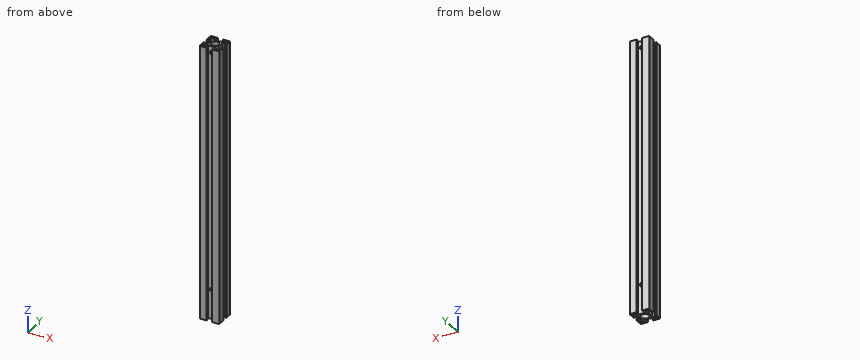
from build123d import *

# Parameters (mm, degrees)
SKETCH006_R     = 6
SKETCH006_W     = 2.75
SKETCH006_H     = 2.75
PAD_DEPTH       = 420
SKETCH_R        = 3.175
POCKET_DEPTH    = 23.250999
SKETCH007_R     = 3.175
POCKET001_DEPTH = 23.251


with BuildPart() as part:
    # Sketch006 → Pad (new body)
    with BuildSketch(Plane.XY):
        with BuildLine():
            Line((4.1, -15), (14, -15))
            ThreePointArc((14, -15), (14.707107, -14.707107), (15, -14))
            Line((15, -14), (15, -4.1))
            Line((15, -4.1), (13, -4.1))
            Line((13, -4.1), (13, -8.75))
            Line((13, -8.75), (11, -8.75))
            Line((11, -8.75), (8.249999, -6))
            Line((8.249999, -6), (8.249999, 6))
            Line((8.249999, 6), (11, 8.75))
            Line((11, 8.75), (13, 8.75))
            Line((13, 8.75), (13, 4.1))
            Line((13, 4.1), (15, 4.1))
            Line((15, 4.1), (15, 14))
            ThreePointArc((15, 14), (14.707107, 14.707107), (14.000001, 15))
            Line((14.000001, 15), (4.1, 15))
            Line((4.1, 15), (4.1, 13))
            Line((4.1, 13), (8.75, 13))
            Line((8.75, 13), (8.75, 11))
            Line((8.75, 11), (6, 8.25))
            Line((6, 8.25), (-6, 8.25))
            Line((-6, 8.25), (-8.75, 11))
            Line((-8.75, 11), (-8.75, 13))
            Line((-8.75, 13), (-4.1, 13))
            Line((-4.1, 13), (-4.1, 15))
            Line((-4.1, 15), (-14, 15))
            ThreePointArc((-14, 15), (-14.707107, 14.707107), (-15, 14))
            Line((-15, 14), (-15, 4.1))
            Line((-15, 4.1), (-13, 4.1))
            Line((-13, 4.1), (-13, 8.75))
            Line((-13, 8.75), (-11, 8.75))
            Line((-11, 8.75), (-8.25, 6))
            Line((-8.25, 6), (-8.25, -6))
            Line((-8.25, -6), (-11, -8.75))
            Line((-11, -8.75), (-13, -8.75))
            Line((-13, -8.75), (-13, -4.1))
            Line((-13, -4.1), (-15, -4.1))
            Line((-15, -4.1), (-15, -14))
            ThreePointArc((-15, -14), (-14.707107, -14.707107), (-14.000001, -15))
            Line((-14.000001, -15), (-4.1, -15))
            Line((-4.1, -15), (-4.1, -13))
            Line((-4.1, -13), (-8.75, -13))
            Line((-8.75, -13), (-8.75, -11))
            Line((-8.75, -11), (-6, -8.249999))
            Line((-6, -8.249999), (6, -8.249999))
            Line((6, -8.249999), (8.75, -11))
            Line((8.75, -11), (8.75, -13))
            Line((8.75, -13), (4.1, -13))
            Line((4.1, -13), (4.1, -15))
        make_face()
        Circle(SKETCH006_R, mode=Mode.SUBTRACT)
        with Locations((-11.625, -11.625)):
            Rectangle(SKETCH006_W, SKETCH006_H, mode=Mode.SUBTRACT)
        with Locations((11.625, -11.625)):
            Rectangle(SKETCH006_W, SKETCH006_H, mode=Mode.SUBTRACT)
        with Locations((11.625, 11.625)):
            Rectangle(SKETCH006_W, SKETCH006_H, mode=Mode.SUBTRACT)
        with Locations((-11.625, 11.625)):
            Rectangle(SKETCH006_W, SKETCH006_H, mode=Mode.SUBTRACT)
    extrude(amount=PAD_DEPTH)

    # Sketch (on Face44 of Pad) → Pocket (cut, through all)
    with BuildSketch(Plane.XZ.offset(8.249999)):
        with Locations((0, 45)):
            Circle(SKETCH_R)
        with Locations((0, 410)):
            Circle(SKETCH_R)
    extrude(amount=-POCKET_DEPTH, mode=Mode.SUBTRACT)

    # Sketch007 (on Face36 of Pocket) → Pocket001 (cut, through all)
    with BuildSketch(Plane(origin=(-8.25, 0, 0), x_dir=(0, -1, 0), z_dir=(-1, 0, 0))):
        with Locations((0, 45)):
            Circle(SKETCH007_R)
        with Locations((0, 410)):
            Circle(SKETCH007_R)
    extrude(amount=-POCKET001_DEPTH, mode=Mode.SUBTRACT)


solid = part.part
Input: part model. Units: mm. Frame: model coordinates. Round coordinates to 2 decimals unless told otherwise and drop trailing zeros.
1) Ray query, L1, parallel to X at y = 12, z = 289.5; L2, parallel to Y at x = 10.5, z = 306.5. Return the intervals inside material, ascending.
2) Contact query for a flat-ended pin moving along its axis: P1, Ø4, axis at y = 0, z = 292.5, coming from the +X side. Output: stop coordinate, or through.
3) Cut plane A-A (z = 316). Count the separate pieces of the cut face and the enclosed holes in it, then the cut area to 3 significant figures.
Geometry says:
1. L1: x = -15 to -13, -10.25 to -8.75, 8.75 to 10.25, 13 to 15
1. L2: y = -15 to -13, -10.25 to -8.25, 8.25 to 10.25, 13 to 15
2. P1: stops at x = 8.25
3. separate pieces: 1
3. enclosed holes: 5
3. area: 388 mm2
